Autodesk Inventor part; units mm, degrees
ref_plane "Work Plane1" through (0, 0, 33.14) normal (0, 0, 1) x (1, 0, 0)
ref_plane "YZ Plane" through (0, 0, 0) normal (1, 0, 0) x (0, 1, 0)
ref_plane "XZ Plane" through (0, 0, 0) normal (0, 1, 0) x (-1, 0, 0)
sketch "Sketch1" plane through (0, 0, 0) normal (0, 0, 1) x (1, 0, 0)
  circle A0 centre (0, 0) radius 1.4605
  dimension "d0" = 2.921
extrude "Extrusion1" add sketch "Sketch1" along normal blind 42.75
ref_plane "Work Plane1" through (0, 0, 33.14) normal (0, 0, 1) x (1, 0, 0)
sketch "Sketch2" plane through (0, 0, 33.14) normal (0, 0, 1) x (1, 0, 0)
  circle A0 centre (0, 0) radius 11.938
  dimension "d5" = 23.876
extrude "Extrusion2" add sketch "Sketch2" against normal blind 8.636
sketch "Sketch3" plane through (0, 0, 24.504) normal (0, 0, -1) x (-1, 0, 0)
  circle A0 centre (0, 0) radius 1.4605
  circle A1 centre (0, 0) radius 10.795
  dimension "d9" = 21.59
extrude "Extrusion3" cut sketch "Sketch3" against normal blind 7.62
properties part number "can"
Can you work these out from the model? Positions are in its coordinate system, mm. A direction names the side the tool comes from. Give positions to 0.01 mm unless a question says otherwise; leave off trailing zeros. Order: outer loops, then holes, each group sorted by start corner. A loop starts at its lowest first (then second) coordinate and runs counter-clockwise, first axis right, second up. Notation, with made-up numbers: M -36.5,35.25 L -23.5,35.25 A23 cw -23.5,58.25 Z; hole C 73,11 d2. An arc over 180 degrees is marked long. Use one line per item in the form item = value. Start each with the question number.
Item 1: Will this pin go through, and if not, where does the flat tip stop? pin 1 Ø1 at (x, y) = (0.5, 2.5) entering from +Z.
Item 2: If we section it at A-A (z = 27): Write out the boundary of the cut face in (x, y) (1 decimal), then the cut area to 3 significant figures.
Item 3: We'd pull the mould along Y, two halves only. Please class faces 1 (the cylindrical face through (-2.588, -11.654, 28.882)), 2 (the flat face through (-3, -11, 24.504)), 3 (the cylindrical face through (7.956, 7.296, 28.261)), 4 (the flat face through (0, -2, 32.124)): +Y half, -Y half, draft (parallel to the pull), parting line (faces both ways), or undercut.
Item 4: For faces 5 (the flat face through (0, 0, 0)), 6 (the cylindrical face through (-0.317, 1.426, 37.878)), which set-ups out of +Z, -Z, +X, -X, +Y, -Y let a thin tool reach every point of the face, with its end or its side?
Item 5: If we section it at D-D (z = 34.5): Write out the boundary of the cut face in (x, y), then the cut area to 3 significant figures.
Item 6: If we section it at C-C (y = 7.5): Write out the boundary of the cut face in (x, z), then the cut area to 3 significant figures.
Item 7: If I drill on line 1 along Y through (x, z) = (0, 27.5) (1 decimal); line 2 along X through (y, z) = (-0.5, 28); line 3 along Z through (x, y) = (6.75, 1.5), over which ranges is the centre line in solid material (lowest first)?
Outcome:
q1.pin_1 = 33.14
q2.outline = C 0,0 d23.9; C 0,0 d2.9; hole C 0,0 d21.6
q2.area = 88.3 mm2
q3.face_1 = parting line
q3.face_2 = draft
q3.face_3 = undercut
q3.face_4 = undercut
q4.face_5 = -Z, +X, -X, +Y, -Y
q4.face_6 = +Z
q5.outline = C 0,0 d2.92
q5.area = 6.70 mm2
q6.outline = M -9.29,24.5 L -7.76,24.5 L -7.76,32.12 L 7.76,32.12 L 7.76,24.5 L 9.29,24.5 L 9.29,33.14 L -9.29,33.14 Z
q6.area = 42.1 mm2
q7.line_1 = -11.9 to -10.8, -1.5 to 1.5, 10.8 to 11.9
q7.line_2 = -11.93 to -10.78, -1.37 to 1.37, 10.78 to 11.93
q7.line_3 = 32.12 to 33.14
